Autodesk Fusion 360 part; units mm, degrees
sketch "Sketch1" plane through (0, 0, 0) normal (0, 1, 0) x (1, 0, 0)
  line L0 (0, 0) -> (50, 0)
  line L1 (50, 0) -> (50, 152.93)
  line L2 (50, 152.93) -> (30, 152.93)
  line L3 (30, 152.93) -> (30, 92.93)
  line L4 (0, 0) -> (0, 72.93)
  line L5 (30, 92.93) -> (20, 92.93)
  line L6 (20, 92.93) -> (0, 72.93)
  circle A0 centre (10, 4.76) radius 2.5
  circle A1 centre (25, 4.76) radius 2.5
  circle A2 centre (40, 4.76) radius 2.5
  line L7 (10, 18.55) -> (40, 18.55) construction
  line L8 (40, 18.55) -> (40, 50.55) construction
  line L9 (40, 50.55) -> (10, 50.55) construction
  line L10 (10, 50.55) -> (10, 18.55) construction
  circle A3 centre (10, 50.55) radius 2.5
  circle A4 centre (40, 50.55) radius 2.5
  circle A5 centre (10, 18.55) radius 2.5
  circle A6 centre (40, 18.55) radius 2.5
  point P0 (10, 50.55)
  dimension "d1" = 50
  dimension "d2" = 152.93
  dimension "d3" = 20
  dimension "d4" = 60
  dimension "d5" = 72.93
  dimension "d6" = 10
  dimension "d16" = 5
  dimension "d17" = 5
  dimension "d18" = 5
  dimension "d19" = 4.76
  dimension "d20" = 10
  dimension "d21" = 4.76
  dimension "d22" = 25
  dimension "d23" = 4.76
  dimension "d24" = 40
  dimension "d33" = 5
  dimension "d34" = 5
  dimension "d35" = 5
  dimension "d36" = 5
  dimension "d37" = 30
  dimension "d38" = 32
  dimension "d39" = 10
  dimension "d40" = 18.55
extrude "Extrude3" add sketch "Sketch1" along normal blind 9
sketch "Sketch4" plane through (30, 0, 0) normal (-1, 0, 0) x (0, 0, 1)
  line L0 (-152.93, 0) -> (-92.93, 0)
  line L1 (-92.93, 0) -> (-92.93, 9)
  line L2 (-92.93, 9) -> (-152.93, 9)
  line L3 (-152.93, 9) -> (-152.93, 0)
  line L4 (-152.93, 4.5) -> (-95, 4.5) construction
  line L5 (-100.93, 9) -> (-100.93, 0) construction
  line L6 (-114.93, 9) -> (-114.93, 0) construction
  line L7 (-128.93, 9) -> (-128.93, 0) construction
  line L8 (-146.93, 9) -> (-146.93, 0) construction
  circle A0 centre (-146.93, 4.5) radius 2.1
  circle A1 centre (-128.93, 4.5) radius 2.1
  circle A2 centre (-114.93, 4.5) radius 2
  circle A3 centre (-100.93, 4.5) radius 2.1
  dimension "d45" = 100.93
  dimension "d46" = 114.93
  dimension "d47" = 128.93
  dimension "d48" = 146.93
  dimension "d49" = 4.2
  dimension "d50" = 4.2
  dimension "d51" = 4
  dimension "d52" = 4.2
hole "Hole2" at (30, 4.5, -146.93) direction (1, 0, 0) diameter 4.2 depth 20 tip angle 118
hole "Hole3" at (30, 4.5, -128.93) direction (1, 0, 0) diameter 4.2 end through all
hole "Hole4" at (30, 4.5, -114.93) direction (1, 0, 0) diameter 4 depth 20 tip angle 118
hole "Hole5" at (30, 4.5, -100.93) direction (1, 0, 0) diameter 4.2 depth 20 tip angle 118
Model file for the job. Use its own axes, mm. A direction names the side the tool comes from. Give positions to 0.01 mm unless a question says otherwise; leave off trailing zeros. Loops run counter-clockwise (first coordinate to the right, second up) from the corner with the lowest first, then second, coordinate; pieces in that order, holes last.
1) Saw through at C-C (z = -4.76). Write the cut outline in (x, y).
2) Pull direction Z, two halves, no side cores. Call faces 1 (the flat face through (10.14, 4.44, -83.07)), 2 (the flat face through (30, 4, -123)), 3 (the cylindrical face through (42.31, 4.44, -19.51)): +Z half, -Z half, draft (parallel to the pull), parting line (faces both ways), or undercut.
3) Saw through at A-A (x = 10). Write the cut outline in (y, z), plus the area to 3 significant figures.
4) Tool access for faces 4 (the flat face through (25, 4, -92.93)), 5 (the cylindrical face through (40.14, 6.55, -129.39)): list every direction of +Z, -Z, +X, -X, +Y, -Y with a clear straight run to the whole face (end or side of a thin tool).
5) Saw through at D-D (z = -114.93). Write the cut outline in (x, y), plus the area to 3 significant figures.
6) Saw through at B-B (y = 4.5). Count the separate pieces of the cut face and the enclosed holes in it, plus the area to 3 significant figures.
7) Flat gauge pins, fed straight in: pin 1 Ø8 at (x, z) = (10, -4.76) entering from +Y; pin 2 Ø4 at (y, z) = (4, -136) entering from -X; pin 3 Ø2.5 at (x, y) = (23.5, 4.5) entering from -Z. Where does each tip first touch, or does it go through?
8) Wall check: line 1 (Z direction, x = 44.5, y = 4.5); line 2 (X direction, y = 6.5, z = -50.55); line 3 (Y direction, x = 42.5, z = -128.93). Give the ranges that are in metal, low to high.
Answer block:
1. outline: (0, 0) - (7.5, 0) - (7.5, 9) - (0, 9) - close; (12.5, 0) - (22.5, 0) - (22.5, 9) - (12.5, 9) - close; (27.5, 0) - (37.5, 0) - (37.5, 9) - (27.5, 9) - close; (42.5, 0) - (50, 0) - (50, 9) - (42.5, 9) - close
2. face 1: -Z half
2. face 2: draft
2. face 3: undercut
3. outline: (0, -82.93) - (9, -82.93) - (9, -53.05) - (0, -53.05) - close; (0, -48.05) - (9, -48.05) - (9, -21.05) - (0, -21.05) - close; (0, -16.05) - (9, -16.05) - (9, -7.26) - (0, -7.26) - close; (0, -2.26) - (9, -2.26) - (9, 0) - (0, 0) - close
3. area: 611 mm2
4. face 4: -Z, -X, +Y, -Y
4. face 5: +X, -X
5. outline: (30, 0) - (50, 0) - (50, 2.5) - (30, 2.5) - close; (30, 6.5) - (50, 6.5) - (50, 9) - (30, 9) - close
5. area: 100 mm2
6. separate pieces: 5
6. enclosed holes: 7
6. area: 5,180 mm2
7. pin 1: stops at y = 9
7. pin 2: stops at x = 30
7. pin 3: stops at z = -92.93
8. line 1: z = -152.93 to -149.03, -144.83 to -131.03, -126.83 to -116.93, -112.93 to -103.03, -98.83 to 0
8. line 2: x = 0 to 7.5, 12.5 to 37.5, 42.5 to 50
8. line 3: y = 0 to 2.4, 6.6 to 9
